Part model, mm, in its own coordinate system. Give positions to 0.01 mm unless a question says otherwise; leave off trailing zeros. Write each loop counter-clockwise with the first axis right and the second up, starting at its lowest first coordinate (ties: lowest second). Pieces come first, ordered by that corner, then holes. Notation, with made-up numbers: M 7.25,86 L 50.25,86 A28 cw 50.25,115 Z; hole C -14,-5.5 d1. An arc over 180 degrees is marked long. Answer as CSV lines item,"result". Start each with the question number.
Item 1: Band-saw the part on A-A, the plane x = 14. List the corners of the cut face in (y, z).
Item 2: Wall check: L1, parallel to Y at x = 61.2, z = 19; L2, parallel to Z at x = 61, y = 21; L3, parallel to Y at x = 60.5, z = 26.75. Give the ranges that are in metal, low to high. Write a range as from..to.
Item 3: Pin check, flat tips, straight feed: pin 1 (8 mm diameter, centred on y = 24.5, z = 20, fed in from -X); pin 2 (2.5 mm diameter, centred on y = 21, z = 34.5, fed in from +X); pin 3 (11.5 mm diameter, centred on x = 38, z = 24, fed in from +Y). Stop position of each tip, or through.
Item 4: Two-plate mould, pull along Z, no slides. Class faces 1 (the flat face through (38, 1, 38)), 2 (the cylindrical face through (61.01, 10.35, 23.76)), 3 (the flat face through (30, 2, 19)): +Z half, -Z half, draft (parallel to the pull), parting line (faces both ways), or undercut.
Item 5: Band-saw the part on C-C, the plane y = 28. List the corners of the cut face in (x, z).
Item 6: Band-saw the part on B-B, the plane z = 26.75. List the corners of the cut face in (x, y), then the cut area to 3 significant figures.
Item 7: Band-saw the part on D-D, the plane z = 4. Count the separate pieces of the cut face and the enclosed holes in it, then the cut area to 3 significant figures.
Autodesk Inventor part; units mm, degrees
ref_plane "YZ Plane" through (0, 0, 0) normal (1, 0, 0) x (0, 1, 0)
ref_plane "XZ Plane" through (0, 0, 0) normal (0, 1, 0) x (-1, 0, 0)
ref_plane "XY Plane" through (0, 0, 0) normal (0, 0, 1) x (1, 0, 0)
sketch "スケッチ1" plane through (0, 0, 0) normal (0, 1, 0) x (-1, 0, 0)
  line L0 (0, 0) -> (-62, 0)
  line L1 (-62, 0) -> (-62, 38)
  line L2 (-62, 38) -> (0, 38)
  line L3 (0, 38) -> (0, 0)
  dimension "d0" = 62
  dimension "d1" = 38
extrude "押し出し1" add sketch "スケッチ1" along normal blind 2
sketch "スケッチ2" plane through (0, 2, 0) normal (0, 1, 0) x (1, 0, 0)
  line L0 (0, 0) -> (0, -38)
  line L1 (62, -38) -> (62, 0)
  line L2 (0, 0) -> (4, 0)
  line L3 (4, 0) -> (4, -4)
  line L4 (4, -4) -> (0, -4)
  line L5 (0, -4) -> (0, 0)
  line L6 (4, -4) -> (14, -4)
  line L7 (14, -4) -> (24, -4)
  line L8 (24, -4) -> (34, -4)
  line L9 (34, -4) -> (44, -4)
  line L10 (44, -4) -> (54, -4)
  line L11 (0, -19) -> (62, -19)
  point P0 (4, -34)
  point P1 (14, -34)
  point P2 (24, -34)
  point P3 (34, -34)
  point P4 (44, -34)
  point P5 (54, -34)
  point P6 (4, -34)
  point P7 (14, -34)
  dimension "d4" = 4
  dimension "d5" = 4
  dimension "d6" = 10
  dimension "d7" = 10
  dimension "d8" = 10
  dimension "d9" = 10
  dimension "d10" = 10
hole "穴1" at (4, 2, 4) at (14, 2, 4) at (24, 2, 4) at (34, 2, 4) at (44, 2, 4) at (54, 2, 4) at (24, 2, 34) at (34, 2, 34) at (44, 2, 34) at (54, 2, 34) at (4, 2, 34) at (14, 2, 34) direction (0, -1, 0) diameter 3 depth 8 tip angle 118
sketch "スケッチ3" plane through (0, 2, 0) normal (0, 1, 0) x (1, 0, 0)
  line L0 (0, -38) -> (62, -38)
  line L1 (62, -38) -> (62, 0)
  line L2 (62, 0) -> (60, 0)
  line L3 (60, 0) -> (60, -38)
  line L4 (60, -38) -> (62, -38)
  line L5 (62, -38) -> (62, 0)
  dimension "d18" = 2
extrude "押し出し2" add sketch "スケッチ3" along normal blind 38
fillet "フィレット1" radius 19 2 edges at (61, 40, 38) (61, 40, 0)
sketch "スケッチ4" plane through (62, 0, 38) normal (1, 0, 0) x (0, 0, -1)
  arc A0 (38, 21) -> (0, 21) centre (19, 21) ccw
  line L0 (38, 0) -> (38, 21)
  circle A1 centre (19, 21) radius 15.5
  circle A2 centre (34.5, 21) radius 1.5
  circle A3 centre (26.75, 34.4234) radius 1.5
  circle A4 centre (11.25, 34.4234) radius 1.5
  circle A5 centre (3.5, 21) radius 1.5
  circle A6 centre (11.25, 7.5766) radius 1.5
  circle A7 centre (26.75, 7.5766) radius 1.5
  line L1 (19, 21) -> (19, 28)
  circle A8 centre (19, 28) radius 6
  line L2 (19, 21) -> (19, 14)
  circle A9 centre (19, 14) radius 6
  dimension "d22" = 31
  dimension "d23" = 3
  dimension "d26" = 360
  dimension "d28" = 7
  dimension "d29" = 12
  dimension "d30" = 7
  dimension "d31" = 12
extrude "押し出し3" cut sketch "スケッチ4" against normal blind 3 contours A1 A2 | A1 A2 | A3 A1 | A1 A3 | A7 A1 | A1 A7 | A4 A1 | A1 A4 | A6 A1 | A1 A6 | A5 A1 | A1 A5 | A8 | A9
properties part number "知能ロボコンタミヤギヤードモータ用マウント"
Output:
1,outline,"M 0,0 L 2,0 L 2,2.5 L 0,2.5 Z; M 0,5.5 L 2,5.5 L 2,32.5 L 0,32.5 Z; M 0,35.5 L 2,35.5 L 2,38 L 0,38 Z"
2,L1,"0..8, 20..22, 34..40"
2,L2,"0..2, 5..33, 36..38"
2,L3,"0..6.08, 9.08..32.92, 35.92..38.35"
3,pin 1,"x = 60"
3,pin 2,"through"
3,pin 3,"y = 2"
4,face 1,"+Z half"
4,face 2,"undercut"
4,face 3,"draft"
5,outline,"M 60,1.34 L 62,1.34 L 62,13 L 60,13 Z; M 60,25 L 62,25 L 62,36.66 L 60,36.66 Z"
6,outline,"M 0,0 L 62,0 L 62,6.08 L 60,6.08 L 60,2 L 0,2 Z; M 60,9.08 L 62,9.08 L 62,32.92 L 60,32.92 Z; M 60,35.92 L 62,35.92 L 62,38.35 L 60,38.35 Z"
6,area,"185 mm²"
7,separate pieces,"8"
7,enclosed holes,"0"
7,area,"144 mm²"
